Design review of the part built by this model. Coordinates are the model's own, in mm. A direction names the side the tool comes from. Coordinates: 2 decimals unless noted, no trailing zeros. Loops run counter-clockwise (first coordinate to the right, second up) from the corner with the lowest first, then second, coordinate; pieces in that order, holes last.
Q1. Wall thickness on probe 1 along X at (y, z) = (14, 42); probe 2 along Y at (x, z) = (-39.5, 50.5); probe 3 along X at (y, z) = (-0.5, 28): over which ranges is each line inside the solid? List them lowest first.
Q2. Add section A-A on x = 12. Give the boundary of the cut face in (y, z), and give its area (3 significant figures).
Q3. Add section B-B on z = 35.5. Give the boundary of the cut face in (x, y).
Q4. Machinability: for faces 1 (the face through (-2, 9, 76.2)), 2 (the face through (-13, -16.5, 21)), which of the approach directions +Z, -Z, +X, -X, +Y, -Y give a long, thin tool a straight path to every point of the face, cutting with its end or side? Answer none if there is none.
Q5. Add section D-D on z = 23. Give the boundary of the cut face in (x, y).
Q6. For P1, Ø5, axis at x = -31.5, z = 65, coming from the -Y side; P2, Ø8, axis at x = -4.5, y = -26.5, coming from the -Z side, all flat-tipped, find the tip position at first contact; note any pin that passes through.
Q7. Add section C-C on y = -9. Give the boundary of the cut face in (x, z).
```python
from build123d import *

# Parameters (mm, degrees)
F0_W     = 93.6522595584
F0_H     = 49.5914518833
F1_DEPTH = 76.2
F2_R     = 16.194136499
F3_DEPTH = 50.8
F4_R     = 21.4719665267
F4_R_2   = 16.194136499
F5_DEPTH = 36.83


with BuildPart() as f1:
    # F0 (on Top) → F1 (new body)
    with BuildSketch(Plane.XY):
        with Locations((-1.5670154244, 8.2959681749)):
            Rectangle(F0_W, F0_H)
    extrude(amount=F1_DEPTH)

    # F2 (on face) → F3 (cut)
    with BuildSketch(Plane.XZ.offset(16.4997577667)):
        with Locations((-2.3752143607, 41.5871702135)):
            Circle(F2_R)
    extrude(amount=-F3_DEPTH, mode=Mode.SUBTRACT)

    # F4 (on face) → F5 (join)
    with BuildSketch(Plane.XZ.offset(16.4997577667)):
        with Locations((-2.3752143607, 41.5871702135)):
            Circle(F4_R)
        with Locations((-2.3752143607, 41.5871702135)):
            Circle(F4_R_2, mode=Mode.SUBTRACT)
    extrude(amount=F5_DEPTH)


solid = f1.part
```
Entries:
1. probe 1: x = -48.39 to -18.56, 13.81 to 45.26
1. probe 2: y = -16.5 to 33.09
1. probe 3: x = -48.39 to -11.19, 6.44 to 45.26
2. outline: (-53.33, 25.64) - (-16.5, 25.64) - (-16.5, 0) - (33.09, 0) - (33.09, 34.13) - (-53.33, 34.13) - close; (-53.33, 49.04) - (33.09, 49.04) - (33.09, 76.2) - (-16.5, 76.2) - (-16.5, 57.54) - (-53.33, 57.54) - close
2. area: 3,660 mm2
3. outline: (-48.39, -16.5) - (-22.97, -16.5) - (-22.97, -53.33) - (-17.38, -53.33) - (-17.38, 33.09) - (-48.39, 33.09) - close; (12.63, -53.33) - (18.22, -53.33) - (18.22, -16.5) - (45.26, -16.5) - (45.26, 33.09) - (12.63, 33.09) - close
4. face 1: +Z, +X, -X, +Y, -Y
4. face 2: -Y
5. outline: (-48.39, -16.5) - (-13.13, -16.5) - (-13.13, -53.33) - (8.37, -53.33) - (8.37, -16.5) - (45.26, -16.5) - (45.26, 33.09) - (-48.39, 33.09) - close
6. P1: stops at y = -16.5
6. P2: stops at z = 20.12
7. outline: (-48.39, 0) - (45.26, 0) - (45.26, 76.2) - (-48.39, 76.2) - close; hole circle Ø32.39 at (-2.38, 41.59)
